Study the drawing (mm; zero at the part's minimum x, y, z) and answer. A direction names the side the tool comes from. Coordinates: 2 decimals unless noted, no trailing zeros. Order: outer loops, then holes, each group sorted by start corner. A loop starts at its lowest first (then second) coordinate and runs counter-clockwise, first axis right, second up.
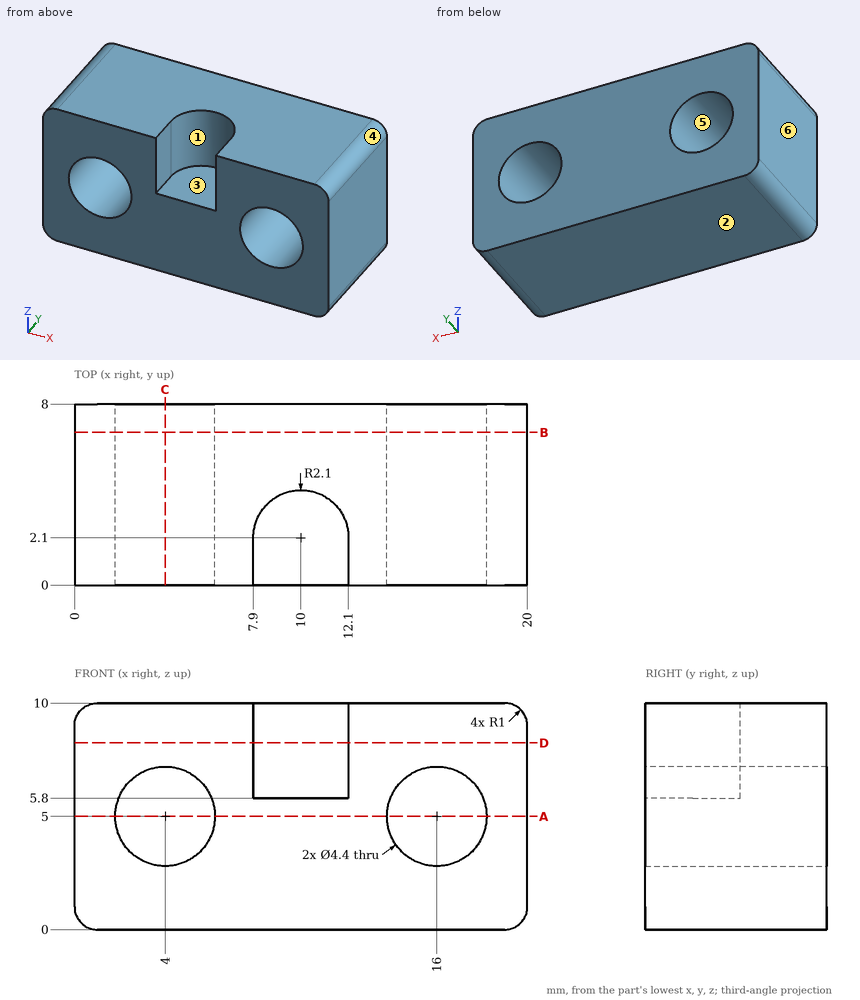
(1) The mould has two halves that part along X. Classify the marked faces 3, 4, 5 and 6: pulls with the +X half, pulls with the -X half, needs draft (parallel to the pull), parting line crosses it, or undercut.
(2) Find section D-D on z = 8.25. Determine the outline of the cut face in (x, y).
(3) Find section C-C on x = 4. Determine the outline of the cut face in (y, z).
(4) Given pin 1 Ø4 at (x, z) = (4, 5) entering from +Y; pin 2 Ø2 at (x, y) = (10, 2.5) entering from +Z, each flat-ended and moving along its own axis, determine where each tip first touches the part or whether it passes through.
(5) Find section A-A on z = 5. Determine the outline of the cut face in (x, y).
(6) A tool of negligible diameter and unlimited length cuts with its end or side. For the marked faces 1 and 2, from which of +Z, -Z, +X, -X, +Y, -Y can it reach the whole face along a straight path? Write none if from no direction.
(7) Find the intervals of material crossed by probe 1 along X at (y, z) = (1.75, 5); probe 2 along X at (y, z) = (5.5, 7); probe 3 along Z at (x, y) = (10.5, 3.5), in increasing order.
(8) Find section B-B on y = 6.75. Determine the outline of the cut face in (x, z), then the cut area to 3 significant figures.
Resolved:
1. face 3: undercut
1. face 4: pulls with the +X half
1. face 5: undercut
1. face 6: pulls with the -X half
2. outline: (0, 0) - (7.9, 0) - (7.9, 2.1) arc R2.1 cw to (12.1, 2.1) - (12.1, 0) - (20, 0) - (20, 8) - (0, 8) - close
3. outline: (0, 0) - (8, 0) - (8, 2.8) - (0, 2.8) - close; (0, 7.2) - (8, 7.2) - (8, 10) - (0, 10) - close
4. pin 1: passes through
4. pin 2: stops at z = 5.8
5. outline: (0, 0) - (1.8, 0) - (1.8, 8) - (0, 8) - close; (6.2, 0) - (13.8, 0) - (13.8, 8) - (6.2, 8) - close; (18.2, 0) - (20, 0) - (20, 8) - (18.2, 8) - close
6. face 1: +Z, -Y
6. face 2: -Z, +X, -X, +Y, -Y
7. probe 1: x = 0 to 1.8, 6.2 to 13.8, 18.2 to 20
7. probe 2: x = 0 to 3.08, 4.92 to 15.08, 16.92 to 20
7. probe 3: z = 0 to 5.8
8. outline: (0, 1) arc R1 ccw to (1, 0) - (19, 0) arc R1 ccw to (20, 1) - (20, 9) arc R1 ccw to (19, 10) - (1, 10) arc R1 ccw to (0, 9) - close; hole circle Ø4.4 at (4, 5); hole circle Ø4.4 at (16, 5)
8. area: 169 mm2
